The model under review builds one solid part; all positions refer to its coordinate system, in mm. A direction names the side the tool comes from. Coordinates: 2 decimals unless noted, no trailing zeros. Order: outer loops, then holes, each group sorted by start corner. A loop starts at its lowest first (then second) coordinate and runs counter-clockwise, first axis right, second up. Notation, with made-up numbers: (65.5, 34.5) -> (95.5, 34.5) arc R15 ccw to (95.5, 61.5) -> close; hole circle Ø4 at (10.5, 15). An arc over 180 degrees is marked (long way). Use one line per item in the form item = value.
from build123d import *

# Parameters (mm, degrees)
F1_DEPTH = 105
F2_R     = 0.25
F3_R     = 2
F3_R_2   = 4.5
F4_DEPTH = 25


with BuildPart() as f1:
    # F0 (on Top) → F1 (new body)
    with BuildSketch(Plane.XY):
        Polygon((-30.083321, 4.672126), (-30.083321, -5.5), (-18.083321, -5.5), (-18.083321, -3.5), (-13.083321, -3.5), (-13.083321, -5.5), (2.916679, -5.5), (2.916679, -3.5), (7.916679, -3.5), (7.916679, -5.5), (19.916679, -5.5), (19.916679, 17.5), (17.916679, 17.5), (17.916679, -3.5), (10.916679, -3.5), (10.916679, 0), (9.393476, 0), (9.393476, -1), (9.893476, -1), (9.893476, -1.5), (5.893476, -1.5), (5.893476, -1), (6.393476, -1), (6.393476, 0), (4.561732, 0), (4.561732, -1), (5.061732, -1), (5.061732, -1.5), (1.061732, -1.5), (1.061732, -1), (1.561732, -1), (1.561732, 0), (-0.083321, 0), (-0.083321, -3.5), (-10.083321, -3.5), (-10.083321, 0), (-11.341457, 0), (-11.341457, -1), (-10.841457, -1), (-10.841457, -1.5), (-14.841457, -1.5), (-14.841457, -1), (-14.341457, -1), (-14.341457, 0), (-16.666559, 0), (-16.666559, -1), (-16.166559, -1), (-16.166559, -1.5), (-20.166559, -1.5), (-20.166559, -1), (-19.666559, -1), (-19.666559, 0), (-21.083321, 0), (-21.083321, -3.5), (-28.083321, -3.5), (-28.083321, 2.672126), (-26.083321, 2.672126), (-26.083321, 4.672126), align=None)
    extrude(amount=F1_DEPTH)

    # F2
    f2_edges = [f1.edges().sort_by_distance(p)[0] for p in [
        (-21.083321, 0, 52.5),
        (-30.083321, 4.672126, 52.5),
        (-26.083321, 4.672126, 52.5),
        (-19.666559, 0, 52.5),
        (-16.666559, 0, 52.5),
        (-14.341457, 0, 52.5),
        (-11.341457, 0, 52.5),
        (-10.083321, 0, 52.5),
        (-0.083321, 0, 52.5),
        (1.561732, 0, 52.5),
        (4.561732, 0, 52.5),
        (6.393476, 0, 52.5),
        (9.393476, 0, 52.5),
        (10.916679, 0, 52.5),
        (17.916679, 17.5, 52.5),
        (-30.083321, -5.5, 52.5),
        (19.916679, 17.5, 52.5),
        (10.916679, -3.5, 52.5),
        (17.916679, -3.5, 52.5),
        (19.916679, -5.5, 52.5),
        (2.916679, -5.5, 52.5),
        (7.916679, -5.5, 52.5),
        (-13.083321, -5.5, 52.5),
        (-18.083321, -5.5, 52.5),
        (-18.083321, -3.5, 52.5),
        (-13.083321, -3.5, 52.5),
        (2.916679, -3.5, 52.5),
        (7.916679, -3.5, 52.5),
    ]]
    fillet(f2_edges, radius=F2_R)

    # F3 (on face) → F4 (cut)
    with BuildSketch(Plane(origin=(0, -3.5, 0), x_dir=(-1, 0, 0), z_dir=(0, 1, 0))):
        with Locations((5.083321, 92.5)):
            Circle(F3_R)
        with Locations((5.083321, 12.5)):
            Circle(F3_R)
        with Locations((5.083321, 52.5)):
            Circle(F3_R_2)
    extrude(amount=-F4_DEPTH, mode=Mode.SUBTRACT)


solid = f1.part
Item 1: Clearance check with flat-ended pins moving along their axes: pin 1 (0.9 mm diameter, centred on x = 1, z = 75.5, fed in from +Y); pin 2 (0.6 mm diameter, centred on x = 5, z = 56.5, fed in from -Y); pin 3 (10 mm diameter, centred on y = 10.5, z = 86.5, fed in from -X). State where each tip first meets the part, or that it passes through.
Results found:
pin_1 = 0
pin_2 = -3.5
pin_3 = 17.92
Item 2: Draft analysis for pull direction Y (two halves, no side actions). For faces 1 (the face through (-18, -1.5, 52)), 2 (the face through (14, -3.5, 52)), 3 (the face through (-3, -4, 0)), state which applies: released by +Y, released by -Y, zero draft, split by the parting line, or undercut.
Results found:
face_1 = undercut
face_2 = released by +Y
face_3 = zero draft
Item 3: Tool access review of faces 4 (the face through (-28.083, 0, 52)), 5 (the face through (-28, 4.672, 52)), 6 (the face through (10.917, -2, 52)): name each direction out of +Z, -Z, +X, -X, +Y, -Y from which nothing blocks a thin tool from reaching the whole face with its end or side.
Results found:
face_4 = +Z, -Z
face_5 = +Z, -Z, -X, +Y
face_6 = +Z, -Z, +Y
Item 4: We need section A-A (x = -25). Write out the cut boundary in (y, z), plus the area to 3 significant figures.
Results found:
outline = (-5.5, 0) -> (-3.5, 0) -> (-3.5, 105) -> (-5.5, 105) -> close
area = 210 mm²
Item 5: We need section B-B (y = 15.5). Write out the cut boundary in (x, z), plus the area to 3 significant figures.
Results found:
outline = (17.92, 0) -> (19.92, 0) -> (19.92, 105) -> (17.92, 105) -> close
area = 210 mm²
Item 6: To check wall thickness, follow L1, parallel to X at y = -1.75, z = 4; L2, parallel to X at y = 1.5, z = 64; L3, parallel to X at y = 4.25, z = 33. State the ranges of each line that lie inside material, in increasing order. Write a range as from..to.
Results found:
L1 = -30.08..-28.08, -21.08..-10.08, -0.08..10.92, 17.92..19.92
L2 = -30.08..-28.08, 17.92..19.92
L3 = -30.08..-26.08, 17.92..19.92
